Source: CAD feature listing. Evaluate the final solid. Frame: model axes, mm. A direction names the side the tool comes from. Round coordinates to 2 decimals unless told otherwise and drop trailing zeros. Loops run counter-clockwise (first coordinate to the right, second up) from the corner with the lowest first, then second, coordinate; pieces in that order, holes last. Notation, with made-up numbers: (78.5, 63.5) -> (111.5, 63.5) arc R16 cw to (111.5, 83.5) -> close; hole circle Ø1 at (75, -33). An arc over 180 degrees is marked (long way). Put each result on its own line as item: value. Start each with the question number.
1. Contact query for flat-ended pins moving along their axis: pin 1 (0.8 mm diameter, centred on x = -12, z = 0, fed in from -Y); pin 2 (12 mm diameter, centred on x = 0, z = -6, fed in from +Y); pin 3 (0.5 mm diameter, centred on x = -12, z = -17, fed in from +Y). Output: stop coordinate, or through.
2. Cut plane C-C (z = -1.5). Return the cut outline in (x, y).
3. Cut plane D-D (x = 5.25). Return the cut outline in (y, z).
4. Set-up query: faces 4 (the flat face through (-12, 1.6, 17)), 5 (the flat face through (12, 4, -3)), 6 (the flat face through (0, 3, 18)), 7 (the flat face through (0, 0, 0)), 8 (the flat face through (12.5, 2, 0)). Return all of +Z, -Z, +X, -X, +Y, -Y with unobstructed straight access to the full face (end or side cutting, diameter ignored); none if empty.
5. Material intervals for L1, parallel to Z at x = 11.75, y = 2.5; L2, parallel to Z at x = 10, y = 3.5; L3, parallel to X at y = 3.75, z = 8, sorted ascending.
6. Cut plane A-A (y = 5.5). Return the cut outline in (x, z), then the cut area to 3 significant figures.
7. Cut plane B-B (y = 3.75). Return the cut outline in (x, z).
8. Draft query along Z for faces 1 (the flat face through (12, 1.6, -17)), 2 (the flat face through (-0.2, 6.4, 18.5)), 3 (the flat face through (0, 3, 19)). Return one class per face: pulls with the +Z half, pulls with the -Z half, needs draft (parallel to the pull), parting line crosses it, or undercut.
```python
from build123d import *

# Parameters (mm, degrees)
SKETCH1_W               = 25
SKETCH1_H               = 38
BOSS_EXTRUDE1_DEPTH     = 6.4
SKETCH2_W               = 23
SKETCH2_H               = 36
CUT_EXTRUDE1_DEPTH      = 6
SKETCH2_3_W             = 1
SKETCH2_3_H             = 1.5
CUT_EXTRUDE2_DEPTH      = 4.8
CUT_EXTRUDE3_DEPTH      = 24.626468208
CUT_EXTRUDE3_DEPTH_BACK = 24.626468208
SKETCH3_W               = 6
SKETCH3_H               = 1.2


with BuildPart() as part:
    # Sketch1 → Boss-Extrude1 (new body)
    with BuildSketch(Plane(origin=(0, 0, 0), x_dir=(1, 0, 0), z_dir=(0, 1, 0))):
        Rectangle(SKETCH1_W, SKETCH1_H)
    extrude(amount=BOSS_EXTRUDE1_DEPTH)

    # Sketch2 → Cut-Extrude1 (cut)
    with BuildSketch(Plane(origin=(0, 6.4, 0), x_dir=(1, 0, 0), z_dir=(0, 1, 0))):
        Rectangle(SKETCH2_W, SKETCH2_H)
    extrude(amount=-CUT_EXTRUDE1_DEPTH, mode=Mode.SUBTRACT)

    # Sketch2_3 → Cut-Extrude2 (cut)
    with BuildSketch(Plane(origin=(0, 6.4, 0), x_dir=(1, 0, 0), z_dir=(0, 1, 0))):
        with Locations((-12, 17.25)):
            Rectangle(SKETCH2_3_W, SKETCH2_3_H)
        with Locations((12, 17.25)):
            Rectangle(SKETCH2_3_W, SKETCH2_3_H)
        with Locations((-12, -17.25)):
            Rectangle(SKETCH2_3_W, SKETCH2_3_H)
        with Locations((12, -17.25)):
            Rectangle(SKETCH2_3_W, SKETCH2_3_H)
    extrude(amount=-CUT_EXTRUDE2_DEPTH, mode=Mode.SUBTRACT)

    # Sketch3 → Cut-Extrude3 (cut, two sides: drawn at the far end of the back side and taken through both)
    with BuildSketch(Plane(origin=(0, 0, 0), x_dir=(0, 0, -1), z_dir=(1, 0, 0)).offset(-CUT_EXTRUDE3_DEPTH_BACK)):
        with Locations((0, 3.6)):
            Rectangle(SKETCH3_W, SKETCH3_H)
    extrude(amount=CUT_EXTRUDE3_DEPTH + CUT_EXTRUDE3_DEPTH_BACK, mode=Mode.SUBTRACT)


solid = part.part
```
Solution:
1. pin 1: stops at y = 0
1. pin 2: stops at y = 0.4
1. pin 3: stops at y = 1.6
2. outline: (-12.5, 0) -> (12.5, 0) -> (12.5, 3) -> (11.5, 3) -> (11.5, 0.4) -> (-11.5, 0.4) -> (-11.5, 3) -> (-12.5, 3) -> close; (-12.5, 4.2) -> (-11.5, 4.2) -> (-11.5, 6.4) -> (-12.5, 6.4) -> close; (11.5, 4.2) -> (12.5, 4.2) -> (12.5, 6.4) -> (11.5, 6.4) -> close
3. outline: (0, -19) -> (6.4, -19) -> (6.4, -18) -> (0.4, -18) -> (0.4, 18) -> (6.4, 18) -> (6.4, 19) -> (0, 19) -> close
4. face 4: +X, -X, +Y
4. face 5: +X, -X
4. face 6: +Y
4. face 7: +Z, -Z, +X, -X, -Y
4. face 8: +Z, -Z, +X, +Y, -Y
5. L1: z = -19 to -18, -16.5 to 16.5, 18 to 19
5. L2: z = -19 to -18, 18 to 19
5. L3: x = -12.5 to -11.5, 11.5 to 12.5
6. outline: (-12.5, -19) -> (12.5, -19) -> (12.5, -18) -> (-12.5, -18) -> close; (-12.5, -16.5) -> (-11.5, -16.5) -> (-11.5, 16.5) -> (-12.5, 16.5) -> close; (-12.5, 18) -> (12.5, 18) -> (12.5, 19) -> (-12.5, 19) -> close; (11.5, -16.5) -> (12.5, -16.5) -> (12.5, 16.5) -> (11.5, 16.5) -> close
6. area: 116 mm^2
7. outline: (-12.5, -19) -> (12.5, -19) -> (12.5, -18) -> (-12.5, -18) -> close; (-12.5, -16.5) -> (-11.5, -16.5) -> (-11.5, -3) -> (-12.5, -3) -> close; (-12.5, 3) -> (-11.5, 3) -> (-11.5, 16.5) -> (-12.5, 16.5) -> close; (-12.5, 18) -> (12.5, 18) -> (12.5, 19) -> (-12.5, 19) -> close; (11.5, -16.5) -> (12.5, -16.5) -> (12.5, -3) -> (11.5, -3) -> close; (11.5, 3) -> (12.5, 3) -> (12.5, 16.5) -> (11.5, 16.5) -> close
8. face 1: undercut
8. face 2: needs draft
8. face 3: pulls with the +Z half
